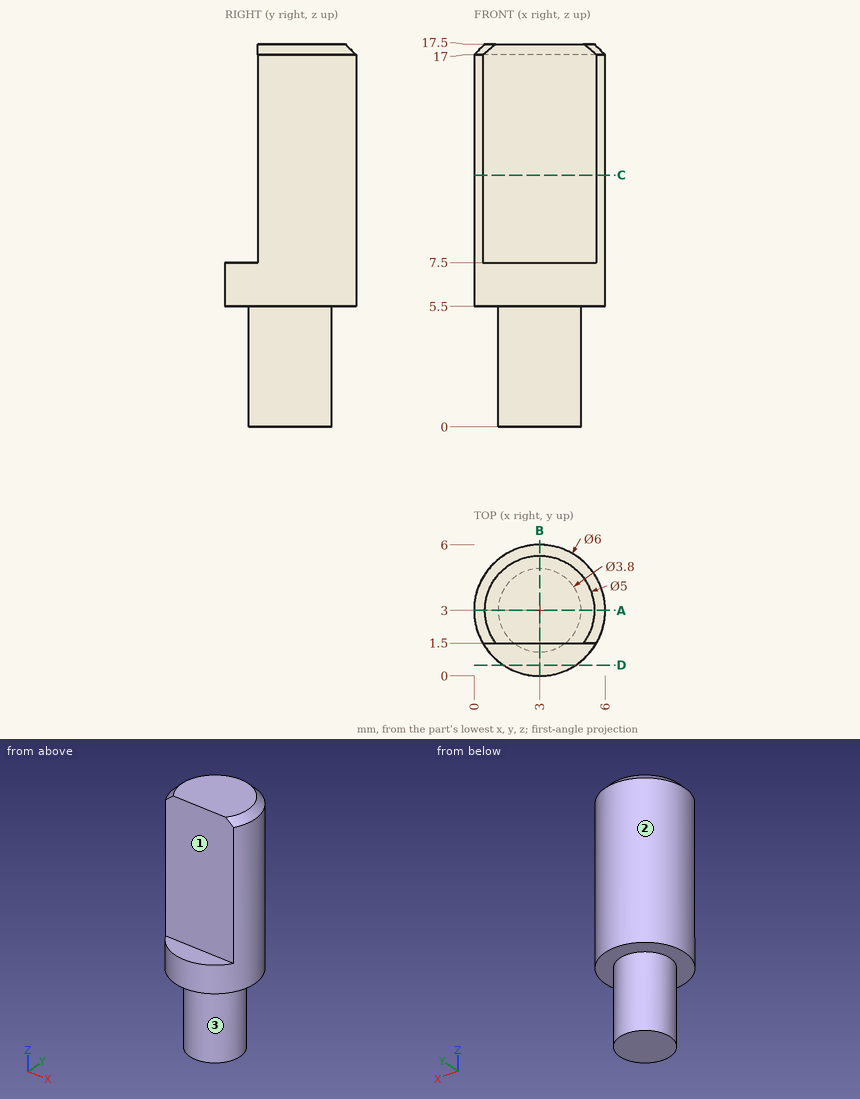
Here's the drawing with two shaded views (mm, measured from the low corner). I have some questions. A direction names the side the tool comes from. Give positions to 0.01 mm unless a question says otherwise; leave off trailing zeros. Write each loop counter-clockwise with the first axis right and the second up, starting at its lowest first coordinate (ties: lowest second). Pieces come first, ordered by that corner, then holes. Notation, with made-up numbers: (-7.75, -15.75) - (8.25, -15.75) arc R22 cw to (8.25, 20.25) - close; hole circle Ø8 at (63.25, 64). An arc over 180 degrees is marked (long way). Write item = value, one per line. Start each with the question number.
1. Imagine slicing it at D-D (y = 0.5). Please give me the cut outline in (x, z), and give its area (3 significant figures).
2. Imagine slicing it at B-B (x = 3). Please give me the cut outline in (y, z), and give its area (3 significant figures).
3. For pin 1 (2 mm diameter, centred on x = 1, z = 4, fed in from -Y); pin 2 (0.5 mm diameter, centred on x = 2.5, y = 0.5, fed in from +Z); pin 3 (2 mm diameter, centred on x = 3, z = 4, fed in from -Y); pin 4 (3 mm diameter, centred on x = 4, y = 3, fed in from -Z), each with a flat end and sliding along its axis, tell me the tip position at first contact or that it passes through.
4. Please list where these lines run through material, in increasing order: line 1 (Z direction, x = 5.2, y = 2.4); line 2 (X direction, y = 3.05, z = 4); line 3 (X direction, y = 4.5, z = 16).
5. Imagine slicing it at A-A (y = 3). Please give me the cut outline in (x, z), and give its area (4 significant figures).
6. Imagine slicing it at C-C (z = 11.5). Please give me the cut outline in (x, y).
7. On a 3-axis mill with a long thin cutter (end or side, diameter ignored), from which of +Z, -Z, +X, -X, +Y, -Y can I reach the whole of each face in a straight line? I mean the marked faces 1, 2 and 3. Say none if no direction works.
Worked answers:
q1.outline = (1.34, 5.5) - (4.66, 5.5) - (4.66, 7.5) - (1.34, 7.5) - close
q1.area = 6.63 mm2
q2.outline = (0, 5.5) - (1.1, 5.5) - (1.1, 0) - (4.9, 0) - (4.9, 5.5) - (6, 5.5) - (6, 17) - (5.5, 17.5) - (1.5, 17.5) - (1.5, 7.5) - (0, 7.5) - close
q2.area = 77.8 mm2
q3.pin_1 = 1.38
q3.pin_2 = 7.5
q3.pin_3 = 1.1
q3.pin_4 = 0
q4.line_1 = 5.5 to 17.5
q4.line_2 = 1.1 to 4.9
q4.line_3 = 0.4 to 5.6
q5.outline = (0, 5.5) - (1.1, 5.5) - (1.1, 0) - (4.9, 0) - (4.9, 5.5) - (6, 5.5) - (6, 17) - (5.5, 17.5) - (0.5, 17.5) - (0, 17) - close
q5.area = 92.65 mm2
q6.outline = (0.4, 1.5) - (5.6, 1.5) arc R3 ccw (long way) to start
q7.face_1 = +Z, +X, -X, -Y
q7.face_2 = +Z, -Z
q7.face_3 = -Z
